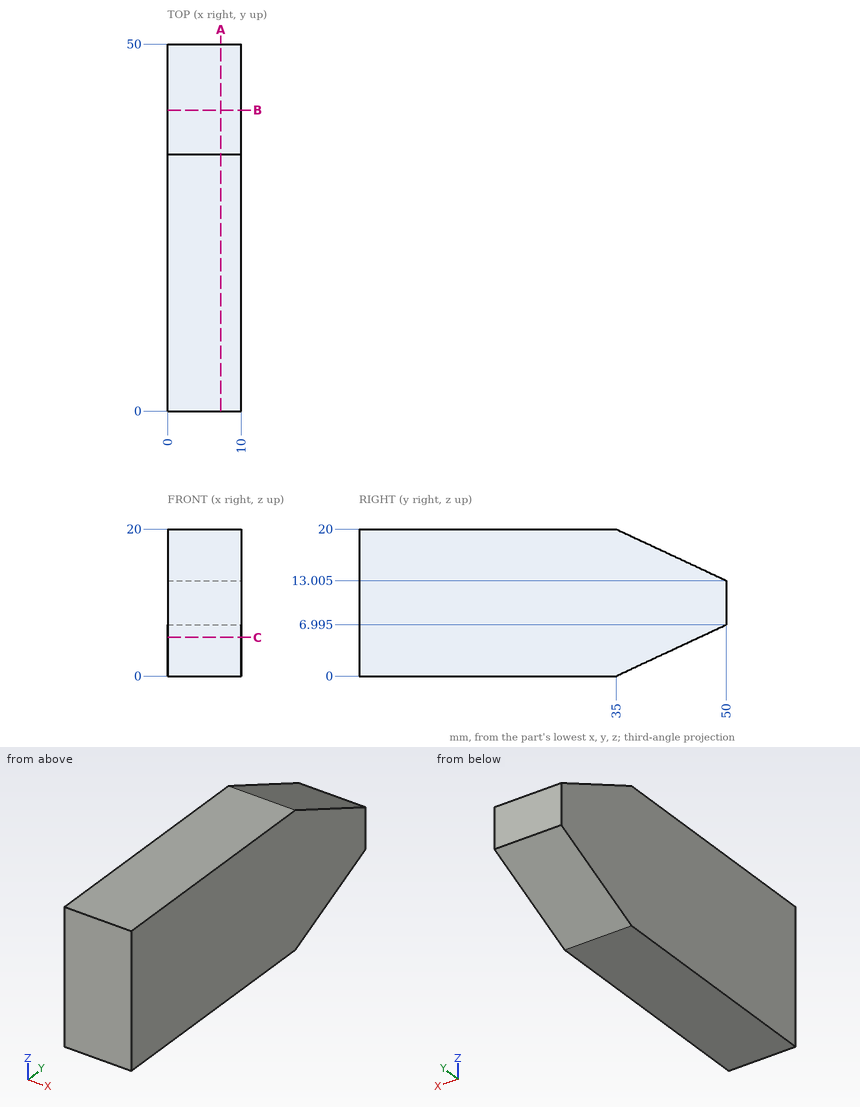
The figure shows three views and two pictorial views of one solid part (mm, origin at its lowest corner). Answer the questions. Round coordinates to 2 decimals unless told otherwise and drop trailing zeros. Write each loop counter-clockwise with the first axis right and the second up, starting at its lowest first coordinate (ties: lowest second). Pieces come first, ordered by that corner, then holes. Notation, with made-up numbers: (22.25, 33) - (76.25, 33) arc R14 cw to (76.25, 41) - close; hole circle Ø8 at (31.25, 16). An arc over 180 degrees is marked (long way). Answer in a Markdown table with one row per item. Add a question column.
1. Given pin 1 (6 mm diameter, centred on x = 5, z = 3.5, fed in from +Y); pin 2 (5 mm diameter, centred on x = 1, z = 2, fed in from +Y), each flat-ended and moving along its own axis, determine where each tip first touches the part or whether it passes through.
2. A cutting plane is placed at A-A, the plane x = 7.25. Determine the outline of the cut face in (y, z) (1 decimal).
3. Find the intervals of material crossed by line 1 along Y through (x, z) = (8.25, 1.25); line 2 along Y through (x, z) = (4.5, 4) (1 decimal); line 3 along Z through (x, y) = (6, 47) (1 decimal), in increasing order. Write a range as from..to.
4. A cutting plane is placed at B-B, the plane y = 41. Determine the outline of the cut face in (x, z).
5. A cutting plane is placed at C-C, the plane z = 5.25. Determine the outline of the cut face in (x, y).
Worked out:
| question | item | result |
|---|---|---|
| 1 | pin 1 | y = 48.94 |
| 1 | pin 2 | y = 44.65 |
| 2 | outline | (0, 0) - (35, 0) - (50, 7) - (50, 13) - (35, 20) - (0, 20) - close |
| 3 | line 1 | 0..37.68 |
| 3 | line 2 | 0..43.6 |
| 3 | line 3 | 5.6..14.4 |
| 4 | outline | (0, 2.8) - (10, 2.8) - (10, 17.2) - (0, 17.2) - close |
| 5 | outline | (0, 0) - (10, 0) - (10, 46.26) - (0, 46.26) - close |
